Input: part model. Units: mm. Frame: model coordinates. A direction names the side the tool comes from. Round coordinates to 2 decimals unless told otherwise and drop trailing zeros. Answer as a JSON object with one key per item and string values.
```python
from build123d import *

# Parameters (mm, degrees)
SKETCH_1_W             = 23.5
SKETCH_1_H             = 12
EXTRUDE_1_DEPTH        = 510.5
HOLE_WIZARD_M6_1_D     = 5
HOLE_WIZARD_M6_1_DEPTH = 19
HOLE_WIZARD_M6_1_TIP   = 1.502151548
HOLE_WIZARD_M6_2_D     = 5
HOLE_WIZARD_M6_2_DEPTH = 19
HOLE_WIZARD_M6_2_TIP   = 1.502151548
SKETCH_6_R             = 4.5
CUT_EXTRUDE_1_DEPTH    = 512.600674355
SKETCH_7_R             = 4.5
CUT_EXTRUDE_2_DEPTH    = 512.600674355
HOLE_WIZARD_M4_1_D     = 3.3
HOLE_WIZARD_M4_1_DEPTH = 11.5
HOLE_WIZARD_M4_1_TIP   = 0.991420021


with BuildPart() as part:
    # 草图1 → 凸台-拉伸1 (new, symmetric)
    with BuildSketch(Plane(origin=(0, 0, 0), x_dir=(0, 0, -1), z_dir=(1, 0, 0))):
        Polygon((-15, 15), (-11.5, 15), (-11.5, 13.5), (-11, 13.5), (-11, 12), (-9.5, 12), (-9.5, 15), (-8, 15), (-8, 12.5), (-5, 12.5), (-5, 15), (5, 15), (5, 12.5), (8, 12.5), (8, 15), (9.5, 15), (9.5, 12), (11, 12), (11, 13.5), (11.5, 13.5), (11.5, 15), (15, 15), (15, 8), (12.5, 8), (12.5, 5), (15, 5), (15, -5), (12.5, -5), (12.5, -8), (15, -8), (15, -15), (11.5, -15), (11.5, -13.5), (11, -13.5), (11, -12), (9.5, -12), (9.5, -15), (8, -15), (8, -12.5), (5, -12.5), (5, -15), (-5, -15), (-5, -12.5), (-8, -12.5), (-8, -15), (-9.5, -15), (-9.5, -12), (-11, -12), (-11, -13.5), (-11.5, -13.5), (-11.5, -15), (-15, -15), align=None)
        with BuildLine():
            Line((12, -10.5), (12, -8.5))
            ThreePointArc((12, -8.5), (11.853553391, -8.146446609), (11.5, -8))
            Line((11.5, -8), (-11.5, -8))
            ThreePointArc((-11.5, -8), (-11.853553391, -8.146446609), (-12, -8.5))
            Line((-12, -8.5), (-12, -10.5))
            ThreePointArc((-12, -10.5), (-11.853553391, -10.853553391), (-11.5, -11))
            Line((-11.5, -11), (11.5, -11))
            ThreePointArc((11.5, -11), (11.853553391, -10.853553391), (12, -10.5))
        make_face(mode=Mode.SUBTRACT)
        with BuildLine():
            Line((-11.5, 11), (11.5, 11))
            ThreePointArc((11.5, 11), (11.853553391, 10.853553391), (12, 10.5))
            Line((12, 10.5), (12, 8.5))
            ThreePointArc((12, 8.5), (11.853553391, 8.146446609), (11.5, 8))
            Line((11.5, 8), (-11.5, 8))
            ThreePointArc((-11.5, 8), (-11.853553391, 8.146446609), (-12, 8.5))
            Line((-12, 8.5), (-12, 10.5))
            ThreePointArc((-12, 10.5), (-11.853553391, 10.853553391), (-11.5, 11))
        make_face(mode=Mode.SUBTRACT)
        Rectangle(SKETCH_1_W, SKETCH_1_H, mode=Mode.SUBTRACT)
    extrude(amount=EXTRUDE_1_DEPTH, both=True)

    # M6 螺纹孔1
    with Locations(Plane(origin=(0, -15, 0), x_dir=(-1, 0, 0), z_dir=(0, -1, 0))):
        with Locations((460.5, 0), (445.5, 0), (-133, 0), (-148, 0), (-218, 0), (-233, 0), (-445.5, 0), (-460.5, 0), (262.5, 0), (211.5, 0)):
            Hole(HOLE_WIZARD_M6_1_D / 2, depth=HOLE_WIZARD_M6_1_DEPTH)
            with Locations((0, 0, -(HOLE_WIZARD_M6_1_DEPTH + HOLE_WIZARD_M6_1_TIP / 2))):  # 118° drill point
                Cone(0, HOLE_WIZARD_M6_1_D / 2, HOLE_WIZARD_M6_1_TIP, mode=Mode.SUBTRACT)

    # M6 螺纹孔2
    with Locations(Plane(origin=(0, 0, -15), x_dir=(-1, 0, 0), z_dir=(0, 0, -1))):
        with Locations((460.5, 0), (445.5, 0), (157.5, 0), (142.5, 0), (-445.5, 0), (-460.5, 0)):
            Hole(HOLE_WIZARD_M6_2_D / 2, depth=HOLE_WIZARD_M6_2_DEPTH)
            with Locations((0, 0, -(HOLE_WIZARD_M6_2_DEPTH + HOLE_WIZARD_M6_2_TIP / 2))):  # 118° drill point
                Cone(0, HOLE_WIZARD_M6_2_D / 2, HOLE_WIZARD_M6_2_TIP, mode=Mode.SUBTRACT)

    # 草图6 → 切除-拉伸1 (cut, through all)
    with BuildSketch(Plane(origin=(0, 15, 0), x_dir=(1, 0, 0), z_dir=(0, 1, 0))):
        with Locations(Location((-495.5, 0, 0), (0, 0, 270))):
            Circle(SKETCH_6_R)
        with Locations(Location((78, 0, 0), (0, 0, 270))):
            Circle(SKETCH_6_R)
    extrude(amount=-CUT_EXTRUDE_1_DEPTH, mode=Mode.SUBTRACT)

    # 草图7 → 切除-拉伸2 (cut, through all)
    with BuildSketch(Plane.XY.offset(15)):
        with Locations((-415.5, 0)):
            Circle(SKETCH_7_R)
        with Locations((422.5, 0)):
            Circle(SKETCH_7_R)
    extrude(amount=-CUT_EXTRUDE_2_DEPTH, mode=Mode.SUBTRACT)

    # M4 螺纹孔1
    with Locations(Plane(origin=(0, 0, -15), x_dir=(-1, 0, 0), z_dir=(0, 0, -1))):
        with Locations((343.5, 0)):
            Hole(HOLE_WIZARD_M4_1_D / 2, depth=HOLE_WIZARD_M4_1_DEPTH)
            with Locations((0, 0, -(HOLE_WIZARD_M4_1_DEPTH + HOLE_WIZARD_M4_1_TIP / 2))):  # 118° drill point
                Cone(0, HOLE_WIZARD_M4_1_D / 2, HOLE_WIZARD_M4_1_TIP, mode=Mode.SUBTRACT)


solid = part.part
```
1) Ray query, probe 1 along Z at (x, y) = (-211.5, -12.6); probe 2 along Y at (x, z) = (80.5, -6); probe 3 along Z at (x, y) = (-312.5, -13.25). Return the intervals inside material, ascending.
Output:
{"probe 1": "z = -15 to -11, -9.5 to -8, -5 to -2.5, 2.5 to 5, 8 to 9.5, 11 to 15", "probe 2": "y = -12.5 to -11, -8 to -6, 6 to 8, 11 to 12.5", "probe 3": "z = -15 to -11, -9.5 to -8, -5 to 5, 8 to 9.5, 11 to 15"}
2) Draft query along Z for faces 1 (the face through (510.5, 7, 0)), 2 (the face through (7, 0, 15)), 3 (the face through (7, 8, 0)). Return one class per face: +Z half, -Z half, draft (parallel to the pull), parting line (faces both ways), or undercut.
Output:
{"face 1": "draft", "face 2": "+Z half", "face 3": "undercut"}
3) Contact query for a flat-ended pin moving along its axis: P1, Ø4.5, axis at x = 133, z = 0, coming from the -Y side. Output: stop coordinate, or through.
Output:
{"P1": "stops at y = 6"}
4) Section A-A, the plane x = -23. Count the separate pieces of the cut face and the enclosed holes in it, plus the area to 3 significant figures.
Output:
{"separate pieces": "1", "enclosed holes": "3", "area": "408 mm^2"}
5) Reachability of faces 4 (the face through (7, -11, 0)), 5 (the face through (-510.5, 7, 0)) from +Z, -Z, +X, -X, +Y, -Y: full face, straight path, thin tool, end or side. Return the list, or none.
Output:
{"face 4": "+X, -X", "face 5": "+Z, -Z, -X, +Y, -Y"}
